Job drawing, mm, ordinate dimensions from the low corner. One solid piece. A direction names the side the tool comes from. Give positions to 0.01 mm unless a question says otherwise; leave off trailing zeros. Order: outer loops, then holes, each group sorted by start corner. A loop starts at its lowest first (then second) coordinate and runs counter-clockwise, first axis right, second up. Notation, with made-up numbers: M -7,47.25 L -2,47.25 A16 ccw -2,55.25 Z; hole C 9.5,23 d9. An arc over 180 degrees is marked long. One line per item, written item: value. Start each with the question number.
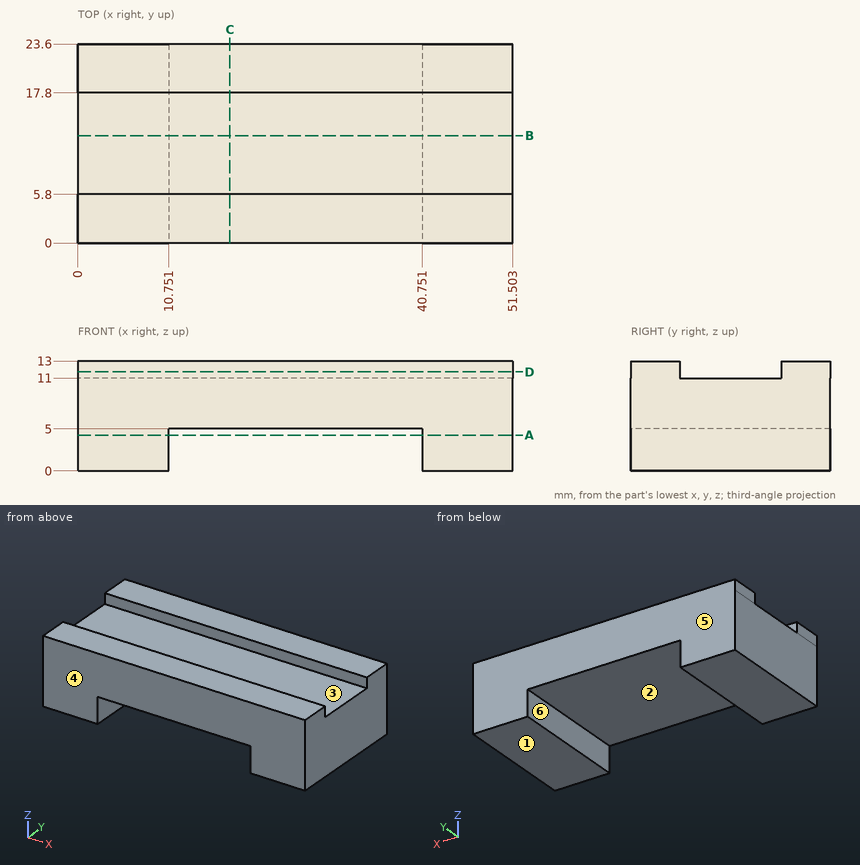
1) Pull direction Y, two halves, no side cores. Call the marked faces 3, 4, 5 and 6: pulls with the +Y half, pulls with the -Y half, needs draft (parallel to the pull), parting line crosses it, or undercut.
2) Slice it at B-B (y = 12.75). List the corners of the cut face in (x, z).
3) Tool access for the marked faces 1 and 2: list every direction of +Z, -Z, +X, -X, +Y, -Y with a clear straight run to the whole face (end or side of a thin tool).
4) Slice it at A-A (z = 4.25). List the corners of the cut face in (x, y).
5) Drill centre lines: line 1 (Y direction, x = 8, z = 11.5); line 2 (Z direction, x = 12.5, y = 11.5); line 3 (X direction, y = 5.5, z = 4.5). Where is each one in solid material? Low to high.
6) Slice it at D-D (z = 11.75). List the corners of the cut face in (x, y).
7) Slice it at C-C (x = 18). List the corners of the cut face in (y, z), plus the area to 3 significant figures.
8) Drop flat-ended pins along their axis: P1, Ø12, axis at x = 26.5, y = 8.5, coming from the -Z side; P2, Ø5, axis at x = 12, y = 11.5, coming from the +Z side. Give the stop position or say it passes through.
Results list:
1. face 3: undercut
1. face 4: pulls with the -Y half
1. face 5: pulls with the +Y half
1. face 6: needs draft
2. outline: M 0,0 L 10.75,0 L 10.75,5 L 40.75,5 L 40.75,0 L 51.5,0 L 51.5,11 L 0,11 Z
3. face 1: -Z, +X, -X, +Y, -Y
3. face 2: -Z, +Y, -Y
4. outline: M 0,0 L 10.75,0 L 10.75,23.6 L 0,23.6 Z; M 40.75,0 L 51.5,0 L 51.5,23.6 L 40.75,23.6 Z
5. line 1: y = 0 to 5.8, 17.8 to 23.6
5. line 2: z = 5 to 11
5. line 3: x = 0 to 10.75, 40.75 to 51.5
6. outline: M 0,0 L 51.5,0 L 51.5,5.8 L 0,5.8 Z; M 0,17.8 L 51.5,17.8 L 51.5,23.6 L 0,23.6 Z
7. outline: M 0,5 L 23.6,5 L 23.6,13 L 17.8,13 L 17.8,11 L 5.8,11 L 5.8,13 L 0,13 Z
7. area: 165 mm²
8. P1: stops at z = 5
8. P2: stops at z = 11
